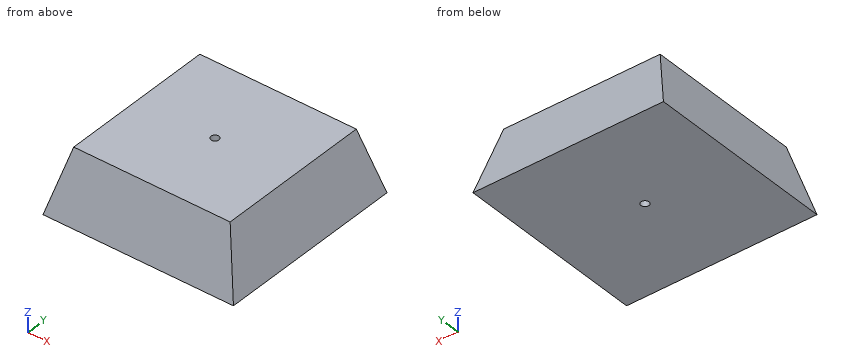
from build123d import *

# Parameters (mm, degrees)
F0_W     = 152.4
F0_H     = 152.4
F0_R     = 3.175
F1_DEPTH = 50.8
F2_SIZE2 = 13.611809
F2_SIZE  = 50.79999


# Not quite as in the source:
# - a fillet or chamfer is up to 0.001 mm smaller than in the source, because OpenCascade refuses the exact size
# - a feature names something its author has since deleted; it is built from what else it names


with BuildPart() as f1:
    # F0 (on Top) → F1 (new body)
    with BuildSketch(Plane.XY):
        with Locations((76.2, 76.2)):
            Rectangle(F0_W, F0_H)
        with Locations((76.2, 76.2)):
            Circle(F0_R, mode=Mode.SUBTRACT)
    extrude(amount=F1_DEPTH)

    # F2 (size 50.8 and 13.6118189755 in the source; OpenCascade refuses exactly that, so slightly less here)
    f2_edges = [f1.edges().sort_by_distance(p)[0] for p in [
        (0, 76.2, 50.8),
        (76.2, 152.4, 50.8),
        (152.4, 76.2, 50.8),
        (76.2, 0, 50.8),
    ]]
    chamfer(f2_edges, length=F2_SIZE, length2=F2_SIZE2)


solid = f1.part
Part model, mm, in its own coordinate system. Round coordinates to 2 decimals unless told otherwise and drop trailing zeros. Write each loop counter-clockwise with the first axis right and the second up, starting at its lowest first coordinate (ties: lowest second). Pieces come first, ordered by that corner, then holes. Notation, with made-up numbers: M 57.25,-39 L 113.25,-39 A18 cw 113.25,-18 Z; hole C -35.75,-17.75 d1. An arc over 180 degrees is marked long. Return JSON: item names as keys, results as strings. Group by question number.
(1) Pin check, flat tips, straight feed: pin 1 Ø6 at (x, z) = (22, 22.5) entering from +Y (3 decimals); pin 2 Ø12 at (x, y) = (47.5, 40.5) entering from -Z; pin 3 Ø12 at (x, z) = (71, 42) entering from +Y; pin 4 Ø12 at (y, z) = (107.5, 44) entering from -X. Stop position of each tip, or through.
(2) Saw through at D-D on z = 18. Write the cut outline in (x, y) (3 decimals).
(3) Drill centre lines: probe 1 along Y at (x, z) = (76.2, 40) (3 decimals); probe 2 along Y at (x, z) = (76, 12); probe 3 along X at (y, z) = (76, 34). Where is each one in solid material? Low to high.
Returned:
{
 "1": {"pin 1": "y = 147.175", "pin 2": "z = 0", "pin 3": "y = 142.75", "pin 4": "x = 10.18"},
 "2": {"outline": "M 4.823,4.823 L 147.577,4.823 L 147.577,147.577 L 4.823,147.577 Z; hole C 76.2,76.2 d6.35"},
 "3": {"probe 1": "10.718 to 73.025, 79.375 to 141.682", "probe 2": "3.22 to 73.03, 79.37 to 149.18", "probe 3": "9.11 to 73.03, 79.37 to 143.29"}
}
